Part model, mm, in its own coordinate system. A direction names the side the tool comes from. Round coordinates to 2 decimals unless told otherwise and drop trailing zeros. Loops run counter-clockwise (first coordinate to the right, second up) from the corner with the lowest first, then second, coordinate; pieces in that order, holes last. Notation, with made-up numbers: (-18, -25) -> (22, -25) arc R20 cw to (22, -10) -> close; hole circle Ø5 at (-39.5, 7). An arc over 180 degrees is marked (long way). Answer as CSV lines item,"result".
from build123d import *

# Parameters (mm, degrees)
F1_DEPTH      = 30
F2_W          = 12
F2_H          = 21.75
F3_DEPTH      = 20.001
F3_DEPTH_BACK = 50.001
F4_R          = 1.9
F5_DEPTH      = 3
F5_DEPTH_BACK = 40.5
F6_DEPTH      = 17.001
F6_DEPTH_BACK = 53.001
F7_W          = 5.1
F7_H          = 5.1
F8_DEPTH      = 2.5


with BuildPart() as f1:
    # F0 (on Front) → F1 (new body, symmetric)
    with BuildSketch(Plane.XZ):
        with BuildLine():
            Line((-35, 0), (0, 0))
            Line((0, 0), (35, 0))
            Line((35, 0), (35, 12.75))
            ThreePointArc((35, 12.75), (34.2195444573, 16.6229833462), (32, 19.8914284285))
            Line((32, 19.8914284285), (32, 26.75))
            Line((32, 26.75), (26.5, 26.75))
            Line((26.5, 26.75), (26.5, 20.3534531629))
            ThreePointArc((26.5, 20.3534531629), (25, 5), (23.5, 20.3534531629))
            Line((23.5, 20.3534531629), (23.5, 26.75))
            Line((23.5, 26.75), (18, 26.75))
            Line((18, 26.75), (18, 19.8914284285))
            ThreePointArc((18, 19.8914284285), (15.7804555427, 16.6229833462), (15, 12.75))
            Line((15, 12.75), (15, 5))
            Line((15, 5), (0, 5))
            Line((0, 5), (-15, 5))
            Line((-15, 5), (-15, 12.75))
            ThreePointArc((-15, 12.75), (-15.7804555427, 16.6229833462), (-18, 19.8914284285))
            Line((-18, 19.8914284285), (-18, 26.75))
            Line((-18, 26.75), (-23.5, 26.75))
            Line((-23.5, 26.75), (-23.5, 20.3534531629))
            ThreePointArc((-23.5, 20.3534531629), (-25, 5), (-26.5, 20.3534531629))
            Line((-26.5, 20.3534531629), (-26.5, 26.75))
            Line((-26.5, 26.75), (-32, 26.75))
            Line((-32, 26.75), (-32, 19.8914284285))
            ThreePointArc((-32, 19.8914284285), (-34.2195444573, 16.6229833462), (-35, 12.75))
            Line((-35, 12.75), (-35, 0))
        make_face()
    extrude(amount=F1_DEPTH, both=True)

    # F2 (on face) → F3 (cut, two sides)
    with BuildSketch(Plane(origin=(15, 0, 0), x_dir=(0, -1, 0), z_dir=(-1, 0, 0))) as f3_sk:
        with Locations((0, 15.875)):
            Rectangle(F2_W, F2_H)
    extrude(amount=-F3_DEPTH, mode=Mode.SUBTRACT)
    extrude(f3_sk.sketch, amount=F3_DEPTH_BACK, mode=Mode.SUBTRACT)

    # F4 (on face) → F5 (cut, two sides)
    with BuildSketch(Plane.YZ.offset(-18)) as f5_sk:
        Polygon((-16.4122867597, 20.3914284285), (-14.8245735195, 23.1414284285), (-16.4122867597, 25.8914284285), (-19.5877132403, 25.8914284285), (-21.1754264805, 23.1414284285), (-19.5877132403, 20.3914284285), align=None)
        with Locations((-18, 23.1414284285)):
            Circle(F4_R, mode=Mode.SUBTRACT)
        Polygon((19.5877132403, 25.8914284285), (16.4122867597, 25.8914284285), (14.8245735195, 23.1414284285), (16.4122867597, 20.3914284285), (19.5877132403, 20.3914284285), (21.1754264805, 23.1414284285), align=None)
        with Locations((18, 23.1414284285)):
            Circle(F4_R, mode=Mode.SUBTRACT)
    extrude(amount=-F5_DEPTH, mode=Mode.SUBTRACT)
    extrude(f5_sk.sketch, amount=F5_DEPTH_BACK, mode=Mode.SUBTRACT)

    # F4 (on face) → F6 (cut, two sides)
    with BuildSketch(Plane.YZ.offset(-18)) as f6_sk:
        with Locations((18, 23.1414284285)):
            Circle(F4_R)
        with Locations((-18, 23.1414284285)):
            Circle(F4_R)
    extrude(amount=-F6_DEPTH, mode=Mode.SUBTRACT)
    extrude(f6_sk.sketch, amount=F6_DEPTH_BACK, mode=Mode.SUBTRACT)

    # F7 (on face) → F8 (cut)
    with BuildSketch(Plane(origin=(0, 0, 0), x_dir=(1, 0, 0), z_dir=(0, 0, -1))):
        with Locations((-12.7, 24.95)):
            Rectangle(F7_W, F7_H)
        with Locations((11.7, 24.95)):
            Rectangle(F7_W, F7_H)
        with Locations((-12.7, 14.97)):
            Rectangle(F7_W, F7_H)
        with Locations((11.7, 14.97)):
            Rectangle(F7_W, F7_H)
        with Locations((-12.7, 4.99)):
            Rectangle(F7_W, F7_H)
        with Locations((11.7, 4.99)):
            Rectangle(F7_W, F7_H)
        with Locations((-12.7, -4.99)):
            Rectangle(F7_W, F7_H)
        with Locations((11.7, -4.99)):
            Rectangle(F7_W, F7_H)
        with Locations((-12.7, -14.97)):
            Rectangle(F7_W, F7_H)
        with Locations((11.7, -14.97)):
            Rectangle(F7_W, F7_H)
        with Locations((-12.7, -24.95)):
            Rectangle(F7_W, F7_H)
        with Locations((11.7, -24.95)):
            Rectangle(F7_W, F7_H)
    extrude(amount=-F8_DEPTH, mode=Mode.SUBTRACT)


solid = f1.part
Q1. Which spindle directions (+Z, -Z, +X, -X, +Y, -Y) get a long thin tool onto all of the face, cutting with end or side? Do faces 4 (the face through (-19.48, -15.63, 21.75)), 5 (the face through (-13, 5, 2.5)), 6 (the face through (18, -21, 24)). Say none if no direction does.
Geometry results:
face 4,"none"
face 5,"-Z"
face 6,"+Z, +Y, -Y"
Q2. Drop flat-ended pins along their axis: P1, Ø2, axis at y = 19, z = 22.5, coming from the -X side; P2, Ø4, axis at y = 22, z = 20.5, coming from the +X side; P3, Ø5, axis at y = 21.5, z = 18.5, coming from the +X side. Give the stop position or say it passes through.
Geometry results:
P1,"x = -32"
P2,"x = 33.18"
P3,"x = 34.46"
Q3. Saw through at D-D, the plane x = 11.5. Write the cut outline in (y, z), then the cut area to 4 significant figures.
Geometry results:
outline,"(-30, 0) -> (-27.5, 0) -> (-27.5, 2.5) -> (-22.4, 2.5) -> (-22.4, 0) -> (-17.52, 0) -> (-17.52, 2.5) -> (-12.42, 2.5) -> (-12.42, 0) -> (-7.54, 0) -> (-7.54, 2.5) -> (-2.44, 2.5) -> (-2.44, 0) -> (2.44, 0) -> (2.44, 2.5) -> (7.54, 2.5) -> (7.54, 0) -> (12.42, 0) -> (12.42, 2.5) -> (17.52, 2.5) -> (17.52, 0) -> (22.4, 0) -> (22.4, 2.5) -> (27.5, 2.5) -> (27.5, 0) -> (30, 0) -> (30, 5) -> (-30, 5) -> close"
area,"223.5 mm2"
Q4. Saw through at A-A, the plane x = -22.5. Write the cut outline in (y, z), then the cut area to 3 significant figures.
Geometry results:
outline,"(-30, 0) -> (30, 0) -> (30, 5.41) -> (6, 5.41) -> (6, 5) -> (-6, 5) -> (-6, 5.41) -> (-30, 5.41) -> close; (-30, 20.09) -> (-6, 20.09) -> (-6, 26.75) -> (-30, 26.75) -> close; (6, 20.09) -> (30, 20.09) -> (30, 26.75) -> (6, 26.75) -> close; hole circle Ø3.8 at (-18, 23.14); hole circle Ø3.8 at (18, 23.14)"
area,"617 mm2"
Q5. Saw through at B-B, the plane z = 14.75. Give the number of separate pieces and of enclosed holes in the cut face, then the cut area to 3 significant figures.
Geometry results:
separate pieces,"8"
enclosed holes,"0"
area,"444 mm2"
Q6. Drill centre lines: line 1 along X through (y, z) = (18.25, 12.75); line 2 along Z through (x, y) = (-28.95, -18); line 3 along X through (y, z) = (16.5, 5.75). Where is each one in solid material? Low to high.
Geometry results:
line 1,"-35 to -32.75, -17.25 to -15, 15 to 17.25, 32.75 to 35"
line 2,"0 to 6.08, 19.42 to 21.24, 25.04 to 26.75"
line 3,"-35 to -28.33, -21.67 to -15, 15 to 21.67, 28.33 to 35"
Q7. Two-plate mould, pull along X, no slides. Class faces 1 (the face through (-0.5, 30, 4.6)), 2 (the face through (-34.2, 17.83, 16.67)), 3 (the face through (20.22, 20.39, 24.5)): pulls with the +X half, pulls with the -X half, needs draft (parallel to the pull), parting line crosses it, or undercut.
Geometry results:
face 1,"needs draft"
face 2,"pulls with the -X half"
face 3,"undercut"
